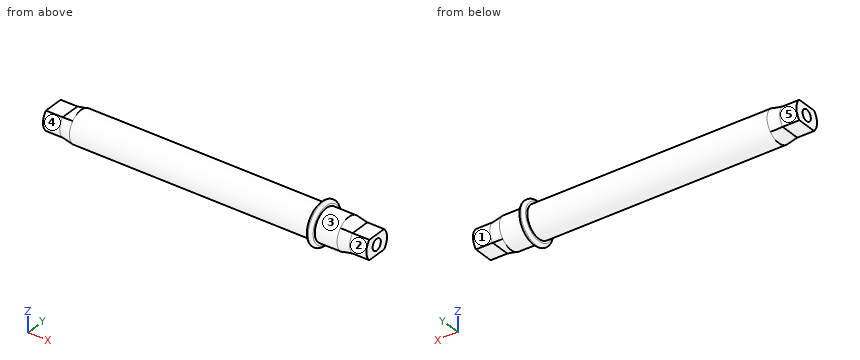
Autodesk Inventor part; units mm, degrees
ref_plane "Work Plane1" through (26, 0, 0) normal (1, 0, 0) x (0, 0, -1)
ref_plane "Work Plane2" through (19, 0, 0) normal (-1, 0, 0) x (0, 0, 1)
ref_plane "YZ Plane" through (0, 0, 0) normal (1, 0, 0) x (0, 1, 0)
sketch "Sketch1" plane through (0, 0, 0) normal (1, 0, 0) x (0, 1, 0)
  circle A0 centre (0, 0) radius 2.85
  dimension "diameter" = 5.7
extrude "Shaft" add sketch "Sketch1" along normal mid plane 48
ref_plane "Work Plane1" through (26, 0, 0) normal (1, 0, 0) x (0, 0, -1)
sketch "Sketch3" plane through (26, 0, 0) normal (1, 0, 0) x (0, 0, -1)
  circle A0 centre (0, 0) radius 2.85 construction
  circle A1 centre (0, 0) radius 2.5
  line L0 (-1.75, 1.7854) -> (1.75, 1.7854)
  line L1 (1.75, 1.7854) -> (1.75, -1.7854)
  line L2 (1.75, -1.7854) -> (-1.75, -1.7854)
  line L3 (-1.75, -1.7854) -> (-1.75, 1.7854)
  line L4 (-1.75, 1.7854) -> (1.75, -1.7854) construction
  line L5 (1.75, 1.7854) -> (-1.75, -1.7854) construction
  dimension "d77" = 5
  dimension "d76" = 3.5
extrude "Wheel Insert Profile" add sketch "Sketch3" along normal blind 3 contours L0 A1 | L1 L2 L3 L0 | A1 L2
loft "Loft1" add section 1 edges at (24, -2.85, 0) section 2 edges at (26, 0, 1.75) (26, 2.5, 0) (26, 0, -1.75) (26, -2.5, 0)
ref_plane "Work Plane2" through (19, 0, 0) normal (-1, 0, 0) x (0, 0, 1)
sketch "Sketch4" plane through (19, 0, 0) normal (-1, 0, 0) x (0, 0, 1)
  circle A0 centre (0, 0) radius 3.75
  dimension "d35" = 7.5
extrude "Stopper" add sketch "Sketch4" against normal blind 1
fillet "Fillet1" radius 0.5 2 edges at (19, 0, -3.75) (20, 0, -3.75)
sketch "Sketch9" plane through (29, 0, 0) normal (1, 0, 0) x (0, 0, -1)
  arc A0 (1.75, 1.7854) -> (-1.75, 1.7854) centre (0, 0) ccw
hole "Hole1" at (29, 0, 0) direction (-1, 0, 0) diameter 2 depth 7
mirror "Mirror1" about plane through (0, 0, 0) normal (1, 0, 0) of "Loft1", "Wheel Insert Profile", "Hole1"
properties part number "front shaft v3"
Check sheet for the modelled part. Datum: model origin and axes. Units: mm. Face numbers are marked on the shaded views. A direction names the side the tool comes from. Round coordinates to 2 decimals unless told otherwise and drop trailing zeros. Write each loop counter-clockwise with the first axis right and the second up, starting at its lowest first coordinate (ties: lowest second). Pieces come first, ordered by that corner, then holes. Notation, with made-up numbers: (-18.5, -21.75) -> (-10.5, -21.75) arc R13 cw to (-10.5, -10.75) -> close; hole circle Ø4 at (25, 23). An arc over 180 degrees is marked (long way). Answer as CSV lines item,"result". Start each with the question number.
1) Material ranges on line 1 (Z direction, x = 26, y = 0); line 2 (Z direction, x = 24, y = 0); line 3 (X direction, y = -0.25, z = 0.75), recorded low to high. Write a range as from..to.
2) Go/stop test with flat-tipped pins: P1, Ø1.8, axis at y = 0, z = 0, coming from the -X side; P2, Ø3, axis at x = 22.5, z = 2.5, coming from the -Y side; P3, Ø3, axis at x = -14, z = 1, coming from the -Y side; P4, Ø1, axis at y = 0.5, z = 0.5, coming from the +X side. Record where each tip stops, or that it passes through.
3) Section check B-B on x = 2.5. Enter the section's corners in (y, z), and give its area (3 significant figures).
4) Tool access check on the marked faces 1, 2, 3, 4 and 5. Record the directions out of +Z, -Z, +X, -X, +Y, -Y that give a thin tool (end or side, any length) a straight path to the whole face; none if there is none.
Found:
1,line 1,"z = -1.75..-1, 1..1.75"
1,line 2,"z = -2.85..-1, 1..2.85"
1,line 3,"x = -22..22"
2,P1,"stops at x = -22"
2,P2,"stops at y = -2.67"
2,P3,"stops at y = -2.85"
2,P4,"stops at x = 29"
3,outline,"circle Ø5.7 at (0, 0)"
3,area,"25.5 mm^2"
4,face 1,"+X, +Y"
4,face 2,"+X, -Y"
4,face 3,"+X"
4,face 4,"-X, -Y"
4,face 5,"-X, +Y"
